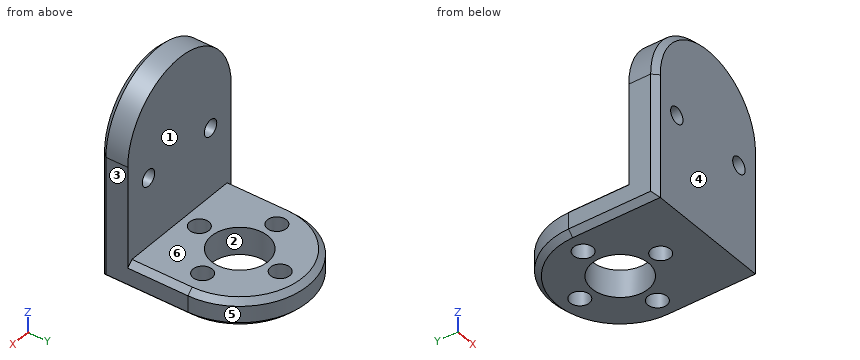
```python
from build123d import *

# Parameters (mm, degrees)
ESQUISSE1_R             = 12.5
ESQUISSE1_R_2           = 5.15
BOSS_EXTRU_1_DEPTH      = 5
BOSS_EXTRU_2_DEPTH      = 5
ESQUISSE3_W             = 25
ESQUISSE3_H             = 5
BOSS_EXTRU_3_DEPTH      = 30
ESQUISSE5_R             = 1.75
ENL_V_MAT_EXTRU_1_DEPTH = 41.462946012
CONG_1_RADIUS           = 12.5
CONG_1_LENGTH           = 5
ESQUISSE6_R             = 1.5
ENL_V_MAT_EXTRU_2_DEPTH = 44.971581732
CHANFREIN1_SIZE         = 1
CHANFREIN2_SIZE         = 1


with BuildPart() as part:
    # Esquisse1 → Boss.-Extru.1 (new body)
    with BuildSketch(Plane.XY):
        Circle(ESQUISSE1_R)
        Circle(ESQUISSE1_R_2, mode=Mode.SUBTRACT)
    extrude(amount=BOSS_EXTRU_1_DEPTH)

    # Esquisse2 → Boss.-Extru.2 (add)
    with BuildSketch(Plane(origin=(0, 0, 0), x_dir=(-1, 0, 0), z_dir=(0, 0, -1))):
        with BuildLine():
            Line((-12.5, 0), (-12.5, -16))
            Line((-12.5, -16), (12.5, -16))
            Line((12.5, -16), (12.5, 0))
            ThreePointArc((12.5, 0), (0, -12.5), (-12.5, 0))
        make_face()
    extrude(amount=-BOSS_EXTRU_2_DEPTH)

    # Esquisse3 → Boss.-Extru.3 (add)
    with BuildSketch(Plane.XY.offset(5)):
        with Locations((0, -13.5)):
            Rectangle(ESQUISSE3_W, ESQUISSE3_H)
    extrude(amount=BOSS_EXTRU_3_DEPTH)

    # Esquisse5 → Enlèv. mat.-Extru.1 (cut, through all)
    with BuildSketch(Plane(origin=(0, 0, 0), x_dir=(-1, 0, 0), z_dir=(0, 0, -1))):
        with Locations((-0.762684291, 7.963561557)):
            Circle(ESQUISSE5_R)
        with Locations((-7.963561557, -0.762684291)):
            Circle(ESQUISSE5_R)
        with Locations((7.963561557, 0.762684291)):
            Circle(ESQUISSE5_R)
        with Locations((0.762684291, -7.963561557)):
            Circle(ESQUISSE5_R)
    extrude(amount=-ENL_V_MAT_EXTRU_1_DEPTH, mode=Mode.SUBTRACT)

    # Congé1: full round fillet: the end face becomes a half cylinder, R = half its width
    cong_1_face = Plane((0, -13.5, 35), x_dir=(0, -1, 0), z_dir=(0, 0, 1))  # on the end face: x along it, z out of the body
    cong_1_slab = cong_1_face.offset(-CONG_1_RADIUS / 2) * Box(CONG_1_LENGTH, 2 * CONG_1_RADIUS, CONG_1_RADIUS, mode=Mode.PRIVATE)  # the body's end, R deep
    cong_1_round = Plane((0, -13.5, 22.5), x_dir=(0, 0, 1), z_dir=(0, -1, 0)) * Cylinder(CONG_1_RADIUS, CONG_1_LENGTH, mode=Mode.PRIVATE)  # its axis R under the face
    add(cong_1_slab - cong_1_round, mode=Mode.SUBTRACT)

    # Esquisse6 → Enlèv. mat.-Extru.2 (cut, through all)
    with BuildSketch(Plane(origin=(0, -11, 0), x_dir=(1, 0, 0), z_dir=(0, 1, 0))):
        with Locations(Location((-7.5, -17.5, 0), (0, 0, 270))):
            Circle(ESQUISSE6_R)
        with Locations(Location((7.5, -17.5, 0), (0, 0, 90))):
            Circle(ESQUISSE6_R)
    extrude(amount=-ENL_V_MAT_EXTRU_2_DEPTH, mode=Mode.SUBTRACT)

    # Chanfrein1
    chanfrein1_edges = [part.edges().sort_by_distance(p)[0] for p in [
        (12.5, -5.5, 5),
        (-12.5, -5.5, 5),
        (0, 12.5, 5),
    ]]
    chamfer(chanfrein1_edges, length=CHANFREIN1_SIZE)

    # Chanfrein2
    chanfrein2_edges = [part.edges().sort_by_distance(p)[0] for p in [
        (12.5, -8, 0),
        (-12.5, -8, 0),
        (0, 12.5, 0),
        (-12.5, -16, 11.25),
        (12.5, -16, 11.25),
        (0, -16, 35),
    ]]
    chamfer(chanfrein2_edges, length=CHANFREIN2_SIZE)


solid = part.part
```
Design review of the part built by this model. Coordinates are the model's own, in mm. Face numbers are marked on the shaded views. A direction names the side the tool comes from. Give positions to 0.01 mm unless a question says otherwise; leave off trailing zeros. Order: outer loops, then holes, each group sorted by start corner. A loop starts at its lowest first (then second) coordinate and runs counter-clockwise, first axis right, second up. Notation, with made-up numbers: (72, 88.25) -> (103, 88.25) arc R15 ccw to (103, 97.25) -> close; hole circle Ø7 at (13, -19). An arc over 180 degrees is marked (long way). Write each question's results on one line, items separated by ' | '. Start each with the question number.
Q1. Wall thickness on L1, parallel to X at y = -12.75, z = 17.5; L2, parallel to X at y = 1.25, z = 4; L3, parallel to Y at x = 0, z = 1.4: over which ranges is each line inside the solid? List them lowest first. Write a range as from..to.
Q2. Add section B-B on z = 2. Give the boundary of the cut face in (x, y).
Q3. Mouldability with a two-part tool opening along Y and no side actions: class the marked faces 1, 2, 3 and 4 as +Y half, -Y half, draft (parallel to the pull), parting line (faces both ways), or undercut.
Q4. Add section C-C on x = 0. Give the boundary of the cut face in (y, z), and give its area (3 significant figures).
Q5. Add section D-D on z = 8. Give the boundary of the cut face in (x, y).
Q6. For pin 1 (5 mm diameter, centred on x = -7.5, z = 17.5, fed in from -Y); pin 2 (8 mm diameter, centred on x = 0, y = 0, fed in from -Z); pin 3 (5.5 mm diameter, centred on x = 7.96, y = -0.76, fed in from +Z); pin 4 (3.5 mm diameter, centred on x = 7.5, z = 17.5, fed in from +Y), all flat-tipped, find the tip position at first contact; note any pin that passes through.
Q7. Machinability: for the marked faces 5 and 6, which of the approach directions +Z, -Z, +X, -X, +Y, -Y give a long, thin tool a straight path to every point of the face, cutting with its end or side? Answer none if there is none.
Q8. Add section A-A on z = 17.5. Give the boundary of the cut face in (x, y), and give its area (3 significant figures).
Found:
1) L1: x = -12.5..-9, -6..6, 9..12.5 | L2: x = -12.44..-9.64, -6.28..-5, 5..12.44 | L3: y = -16..-9.54, -6.39..-5.15, 5.15..6.39, 9.54..12.5
2) outline: (-12.5, -15) -> (-11.5, -16) -> (11.5, -16) -> (12.5, -15) -> (12.5, 0) arc R12.5 ccw to (-12.5, 0) -> close; hole circle Ø3.5 at (-7.96, 0.76); hole circle Ø10.3 at (0, 0); hole circle Ø3.5 at (-0.76, -7.96); hole circle Ø3.5 at (0.76, 7.96); hole circle Ø3.5 at (7.96, -0.76)
3) face 1: +Y half | face 2: undercut | face 3: draft | face 4: -Y half
4) outline: (-16, 0) -> (-9.54, 0) -> (-9.54, 5) -> (-11, 5) -> (-11, 35) -> (-15, 35) -> (-16, 34) -> close; (-6.39, 0) -> (-5.15, 0) -> (-5.15, 5) -> (-6.39, 5) -> close; (5.15, 0) -> (6.39, 0) -> (6.39, 5) -> (5.15, 5) -> close; (9.54, 0) -> (11.5, 0) -> (12.5, 1) -> (12.5, 4) -> (11.5, 5) -> (9.54, 5) -> close | area: 208 mm2
5) outline: (-12.5, -15) -> (-11.5, -16) -> (11.5, -16) -> (12.5, -15) -> (12.5, -11) -> (-12.5, -11) -> close
6) pin 1: stops at y = -16 | pin 2: passes through | pin 3: stops at z = 5 | pin 4: stops at y = -11
7) face 5: +Z, -Z, +Y | face 6: +Z, +X, -X, +Y
8) outline: (-12.5, -15) -> (-11.5, -16) -> (-9, -16) -> (-9, -11) -> (-12.5, -11) -> close; (-6, -16) -> (6, -16) -> (6, -11) -> (-6, -11) -> close; (9, -16) -> (11.5, -16) -> (12.5, -15) -> (12.5, -11) -> (9, -11) -> close | area: 94.0 mm2
